from build123d import *

# Parameters (mm, degrees)
EXTRUDE_2_DEPTH          = 91
FILLET_2_R               = 6
CUT_EXTRUDE_3_DEPTH      = 2.9
CUT_EXTRUDE_3_DEPTH_BACK = 2.9
CUT_EXTRUDE_4_DEPTH      = 2.9
CUT_EXTRUDE_4_DEPTH_BACK = 2.9
CUT_EXTRUDE_5_REACH      = 96.666
SKETCH_17_R              = 1.186185632
SKETCH_17_R_2            = 1.2
CHAMFER_1_SIZE           = 1.2
CUT_EXTRUDE_6_DEPTH      = 91
CUT_EXTRUDE_7_DEPTH      = 96.001094263
CUT_EXTRUDE_7_DEPTH_BACK = 96.001094263


with BuildPart() as part:
    # Эскиз2 → Бобышка-Вытянуть2 (new body)
    with BuildSketch(Plane(origin=(0, 0, 0), x_dir=(0, 0, -1), z_dir=(1, 0, 0))):
        Polygon((-26.444619702, 0), (5.555380298, 0), (5.584037691, -6.7), (-26.444619702, -1.2), align=None)
    extrude(amount=EXTRUDE_2_DEPTH)

    # Скругление2
    fillet_2_edges = [part.edges().sort_by_distance(p)[0] for p in [
        (91, -3.35, -5.569708994),
        (0, -3.35, -5.569708994),
    ]]
    fillet(fillet_2_edges, radius=FILLET_2_R)

    # Эскиз7 → Вырез-Вытянуть3 (cut, two sides: drawn at the far end of the back side and taken through both)
    with BuildSketch(Plane(origin=(22.76798721, 0, -4.425648392), x_dir=(0, -1, 0), z_dir=(0.9816271834476652, 0, -0.19080899537653845)).offset(-CUT_EXTRUDE_3_DEPTH_BACK)):
        Polygon((0, -17.611696981), (0, -24.901696981), (1.7, -25.042701632), (3.07611105, -17.995807395), align=None)
    extrude(amount=CUT_EXTRUDE_3_DEPTH + CUT_EXTRUDE_3_DEPTH_BACK, mode=Mode.SUBTRACT)

    # Эскиз16 → Вырез-Вытянуть4 (cut, two sides: drawn at the far end of the back side and taken through both)
    with BuildSketch(Plane(origin=(64.918878173, 0, 12.618951608), x_dir=(0, -1, 0), z_dir=(-0.9816271834476652, 0, -0.19080899537653845)).offset(-CUT_EXTRUDE_4_DEPTH_BACK)):
        Polygon((0, 0.219393943), (3.063590709, 0.693115345), (1.688216377, 7.740153407), (0, 7.540339831), align=None)
    extrude(amount=CUT_EXTRUDE_4_DEPTH + CUT_EXTRUDE_4_DEPTH_BACK, mode=Mode.SUBTRACT)

    # Вырез-Вытянуть5: up to this plane
    cut_extrude_5_end = Plane(origin=(91, 0, 26.444619702), z_dir=(0, -1, 0))
    # Эскиз17 → Вырез-Вытянуть5 (cut, up to the surface)
    with BuildSketch(Plane(origin=(0, -5.576656818, 0.957630291), x_dir=(1, 0, 0), z_dir=(0, -0.9855741825905647, 0.16924399726708236)), mode=Mode.PRIVATE) as cut_extrude_5_sk1:
        with Locations(Location((88, 7.222581836, 0), (0, 0, 270))):
            Circle(SKETCH_17_R)
    cut_extrude_5_tool1 = split(extrude(cut_extrude_5_sk1.sketch, amount=-CUT_EXTRUDE_5_REACH, mode=Mode.PRIVATE), bisect_by=cut_extrude_5_end, keep=Keep.BOTH, mode=Mode.PRIVATE)
    add(cut_extrude_5_tool1.solids().sort_by_distance((88, -4.354278, 8.07602))[0], mode=Mode.SUBTRACT)
    # Эскиз17 → Вырез-Вытянуть5 (cut, up to the surface)
    with BuildSketch(Plane(origin=(0, -5.576656818, 0.957630291), x_dir=(1, 0, 0), z_dir=(0, -0.9855741825905647, 0.16924399726708236)), mode=Mode.PRIVATE) as cut_extrude_5_sk2:
        with Locations(Location((3, 7.222581836, 0), (0, 0, 270))):
            Circle(SKETCH_17_R_2)
    cut_extrude_5_tool2 = split(extrude(cut_extrude_5_sk2.sketch, amount=-CUT_EXTRUDE_5_REACH, mode=Mode.PRIVATE), bisect_by=cut_extrude_5_end, keep=Keep.BOTH, mode=Mode.PRIVATE)
    add(cut_extrude_5_tool2.solids().sort_by_distance((3, -4.354278, 8.07602))[0], mode=Mode.SUBTRACT)

    # Фаска1
    chamfer_1_edges = [part.edges().sort_by_distance(p)[0] for p in [
        (88, -4.1535234, 9.245094415),
        (3, -4.151185401, 9.258709499),
    ]]
    chamfer(chamfer_1_edges, length=CHAMFER_1_SIZE)

    # Эскиз21 → Вырез-Вытянуть6 (cut)
    with BuildSketch(Plane(origin=(91, 0, 0), x_dir=(0, 0, -1), z_dir=(1, 0, 0))):
        Polygon((-26.444619702, 0), (-26.377093105, -1.211595749), (-26.444619702, -1.2), align=None)
    extrude(amount=-CUT_EXTRUDE_6_DEPTH, mode=Mode.SUBTRACT)

    # Эскиз22 → Вырез-Вытянуть7 (cut, two sides: drawn at the far end of the back side and taken through both)
    with BuildSketch(Plane(origin=(0, 0, 0), x_dir=(1, 0, 0), z_dir=(0, 1, 0)).offset(-CUT_EXTRUDE_7_DEPTH_BACK)):
        with BuildLine():
            ThreePointArc((1.126602828, -26.444619702), (0.288591109, -24.783045247), (0, -22.944619702))
            Line((0, -22.944619702), (0, -26.444619702))
            Line((0, -26.444619702), (1.126602828, -26.444619702))
        make_face()
        with BuildLine():
            ThreePointArc((90.999774909, -22.944972896), (90.711129698, -24.783213348), (89.873172092, -26.444619702))
            Line((89.873172092, -26.444619702), (91, -26.444619702))
            Line((91, -26.444619702), (91, -19.121160447))
            Line((91, -19.121160447), (90.999774909, -22.944972896))
        make_face()
    extrude(amount=CUT_EXTRUDE_7_DEPTH + CUT_EXTRUDE_7_DEPTH_BACK, mode=Mode.SUBTRACT)


solid = part.part
Build history of the part. All positions in model axes, mm. A direction names the side the tool comes from. Round coordinates to 2 decimals unless told otherwise and drop trailing zeros. Write each loop counter-clockwise with the first axis right and the second up, starting at its lowest first coordinate (ties: lowest second). Pieces come first, ordered by that corner, then holes. Notation, with made-up numbers: (45.25, -1) - (100.25, -1) arc R27 cw to (100.25, 30) - close; hole circle Ø10 at (2, -20.5). An arc over 180 degrees is marked (long way). One line per question, with ' | ' between items.
1. Band-saw the part on A-A, the plane x = 35.5. Write the cut outline in (y, z).
Results are:
outline: (-6.7, -5.58) - (0, -5.56) - (0, 26.44) - (-1.21, 26.38) - close
2. Band-saw the part on B-B, the plane z = 7.5. Give the number of separate pieces and of enclosed holes in the cut face, and give its area (3 significant figures).
Results are:
separate pieces: 3 | enclosed holes: 0 | area: 382 mm^2
3. Band-saw the part on D-D, the plane x = 63. Write the cut outline in (y, z).
Results are:
outline: (-6.7, -5.58) - (0, -5.56) - (0, 12.47) - (-3.06, 12.95) - (-1.69, 20.13) - (0, 19.93) - (0, 26.44) - (-1.21, 26.38) - close
4. Band-saw the part on C-C, the plane z = 3. Write the cut outline in (x, y), and give its area (3 significant figures).
Results are:
outline: (0, -5.23) - (91, -5.23) - (91, 0) - (0, 0) - close | area: 476 mm^2
5. Drop flat-ended pins along their axis: pin 1 Ø12 at (x, z) = (65, 21) entering from -Y; pin 2 Ø1.5 at (y, z) = (-5, 18) entering from -X; pin 3 Ø6 at (x, z) = (18.5, 3) entering from -Y. Give the stop position or say it passes through.
Results are:
pin 1: y = -3.17 | pin 2: through | pin 3: y = -5.74
6. Mould opens along Z. For faces 4 (the face through (88.356, -1.701, 6.472)), 5 (the face through (45, 0, 11)), 6 (the face through (26.84, -2.38, 16.75)), 7 (the face through (90.72, -0.71, 24.76)) say: released by +Z, released by -Z, zero draft, split by the parting line, or undercut.
Results are:
face 4: undercut | face 5: zero draft | face 6: undercut | face 7: released by +Z
7. Tool access for faces 1 (the face through (27.493, -0.838, 20.095)), 2 (the face through (0, -2, 9)), 3 (the face through (26.13, -1.56, 13.06)): list every direction of +Z, -Z, +X, -X, +Y, -Y with a clear straight run to the whole face (end or side of a thin tool).
Results are:
face 1: none | face 2: +Z, -Z, -X, +Y, -Y | face 3: +Y
8. Drill centre lines: line 1 along X through (y, z) = (-0.25, 19); line 2 along Y through (x, z) = (7, 15); line 3 along Y through (x, z) = (51.5, 17.5). Where is each one in solid material? Low to high. Write a range as from..to.
Results are:
line 1: 0..24.37, 30.28..60.72, 66.63..91 | line 2: -3.17..0 | line 3: -2.74..0
